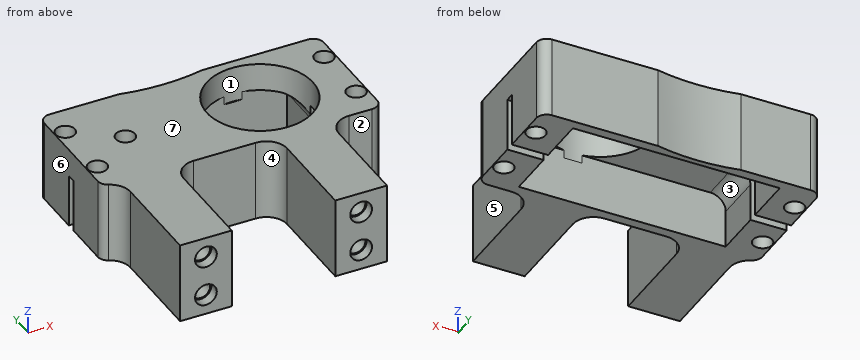
from build123d import *

# Parameters (mm, degrees)
SKETCH035_R                   = 7
SKETCH035_R_2                 = 1.85
PAD021_DEPTH                  = 5.4
PAD021_DEPTH_BACK             = 10.3
POCKET019_DEPTH               = 10.1
SKETCH039_W                   = 1.7
SKETCH039_H                   = 20
POCKET020_DEPTH               = 54.001
SKETCH043_R                   = 10.25
POCKET023_DEPTH               = 7
SKETCH044_W                   = 10
SKETCH044_H                   = 7.85
PAD025_DEPTH                  = 22
SKETCH045_R                   = 1.85
POCKET024_DEPTH               = 12
SKETCH046_R                   = 2.1
POCKET025_DEPTH               = 2
SKETCH044_MIRRORED002_2_W     = 10
SKETCH044_MIRRORED002_2_H     = 7.85
PAD025_MIRRORED002_2_DEPTH    = 22
SKETCH045_MIRRORED002_2_R     = 1.85
POCKET024_MIRRORED002_2_DEPTH = 12
SKETCH046_MIRRORED002_2_R     = 2.1
POCKET025_MIRRORED002_2_DEPTH = 2
FILLET009_R                   = 4


with BuildPart() as part:
    # Sketch035 → Pad021 (new body, two sides)
    with BuildSketch(Plane.XY) as pad021_sk:
        with BuildLine():
            Line((-23.5, 10), (-23.5, -10))
            ThreePointArc((-23.5, -10), (-22.914214, -11.414214), (-21.5, -12))
            Line((-21.5, -12), (28.5, -12))
            ThreePointArc((28.5, -12), (29.914214, -11.414214), (30.5, -10))
            Line((30.5, -10), (30.5, 10))
            ThreePointArc((30.5, 10), (29.914214, 11.414214), (28.5, 12))
            Line((8, 12), (28.5, 12))
            ThreePointArc((-8, 12), (0, 11.167024), (8, 12))
            Line((-21.5, 12), (-8, 12))
            ThreePointArc((-21.5, 12), (-22.914214, 11.414214), (-23.5, 10))
        make_face()
        with Locations((13, 0)):
            Circle(SKETCH035_R, mode=Mode.SUBTRACT)
        with Locations((-21.5, 6)):
            Circle(SKETCH035_R_2, mode=Mode.SUBTRACT)
        with Locations((-21.5, -6)):
            Circle(SKETCH035_R_2, mode=Mode.SUBTRACT)
        with Locations((28.5, 6)):
            Circle(SKETCH035_R_2, mode=Mode.SUBTRACT)
        with Locations((28.5, -6)):
            Circle(SKETCH035_R_2, mode=Mode.SUBTRACT)
        with Locations((-13, 0)):
            Circle(SKETCH035_R_2, mode=Mode.SUBTRACT)
    extrude(amount=PAD021_DEPTH)
    extrude(pad021_sk.sketch, amount=-PAD021_DEPTH_BACK)

    # Sketch038 → Pocket019 (cut, symmetric)
    with BuildSketch(Plane.XZ):
        with BuildLine():
            Line((-16.5, -3), (-16.5, -20))
            Line((-16.5, -20), (23.5, -20))
            Line((23.5, -20), (23.5, -3))
            ThreePointArc((23.5, -3), (22.62132, -0.87868), (20.5, 0))
            Line((20.5, 0), (-13.5, 0))
            ThreePointArc((-13.5, 0), (-15.62132, -0.87868), (-16.5, -3))
        make_face()
    extrude(amount=POCKET019_DEPTH, both=True, mode=Mode.SUBTRACT)

    # Sketch039 (on Face3 of Pocket019) → Pocket020 (cut, through all)
    with BuildSketch(Plane(origin=(-23.5, 0, 0), x_dir=(0, -1, 0), z_dir=(-1, 0, 0))):
        with Locations((0, -10)):
            Rectangle(SKETCH039_W, SKETCH039_H)
    extrude(amount=-POCKET020_DEPTH, mode=Mode.SUBTRACT)

    # Sketch043 (on Face5 of Pocket020) → Pocket023 (cut)
    with BuildSketch(Plane.XY.offset(5.4)):
        with Locations((13, 0)):
            Circle(SKETCH043_R)
    extrude(amount=-POCKET023_DEPTH, mode=Mode.SUBTRACT)

    # Sketch044 → Pad025 (join)
    with BuildSketch(Plane(origin=(0, -12, -2.45), x_dir=(1, 0, 0), z_dir=(0, -1, 0))):
        with Locations((-15, 3.925)):
            Rectangle(SKETCH044_W, SKETCH044_H)
    pad025 = extrude(amount=PAD025_DEPTH)

    # Sketch045 (on Face43 of Pad025) → Pocket024 (cut)
    with BuildSketch(Plane.XZ.offset(34)):
        with Locations((-15, 1.475)):
            Circle(SKETCH045_R)
    pocket024 = extrude(amount=-POCKET024_DEPTH, mode=Mode.SUBTRACT)

    # Sketch046 (on Face43 of Pocket024) → Pocket025 (cut)
    with BuildSketch(Plane.XZ.offset(34)):
        with Locations((-15, 1.475)):
            Circle(SKETCH046_R)
    pocket025 = extrude(amount=-POCKET025_DEPTH, mode=Mode.SUBTRACT)

    # Sketch044 Mirrored002 2 → Pad025 Mirrored002 2 (add)
    with BuildSketch(Plane(origin=(0, -12, -2.45), x_dir=(-1, 0, 0), z_dir=(0, 1, 0))):
        with Locations((-15, 3.925)):
            Rectangle(SKETCH044_MIRRORED002_2_W, SKETCH044_MIRRORED002_2_H)
    pad025_mirrored002_2 = extrude(amount=-PAD025_MIRRORED002_2_DEPTH)

    # Sketch045 Mirrored002 2 → Pocket024 Mirrored002 2 (cut)
    with BuildSketch(Plane(origin=(0, -34, 0), x_dir=(-1, 0, 0), z_dir=(0, 1, 0))):
        with Locations((-15, 1.475)):
            Circle(SKETCH045_MIRRORED002_2_R)
    pocket024_mirrored002_2 = extrude(amount=POCKET024_MIRRORED002_2_DEPTH, mode=Mode.SUBTRACT)

    # Sketch046 Mirrored002 2 → Pocket025 Mirrored002 2 (cut)
    with BuildSketch(Plane(origin=(0, -34, 0), x_dir=(-1, 0, 0), z_dir=(0, 1, 0))):
        with Locations((-15, 1.475)):
            Circle(SKETCH046_MIRRORED002_2_R)
    pocket025_mirrored002_2 = extrude(amount=POCKET025_MIRRORED002_2_DEPTH, mode=Mode.SUBTRACT)

    # Mirrored003: Pad025, Pocket024, Pocket025, Pad025 Mirrored002 2, Pocket024 Mirrored002 2, Pocket025 Mirrored002 2 across Sketch044 H_Axis
    add(pad025.mirror(Plane(origin=(0, -12, -2.45), x_dir=(0, -1, 0), z_dir=(0, 0, 1))))
    add(pocket024.mirror(Plane(origin=(0, -12, -2.45), x_dir=(0, -1, 0), z_dir=(0, 0, 1))), mode=Mode.SUBTRACT)
    add(pocket025.mirror(Plane(origin=(0, -12, -2.45), x_dir=(0, -1, 0), z_dir=(0, 0, 1))), mode=Mode.SUBTRACT)
    add(pad025_mirrored002_2.mirror(Plane(origin=(0, -12, -2.45), x_dir=(0, -1, 0), z_dir=(0, 0, 1))))
    add(pocket024_mirrored002_2.mirror(Plane(origin=(0, -12, -2.45), x_dir=(0, -1, 0), z_dir=(0, 0, 1))), mode=Mode.SUBTRACT)
    add(pocket025_mirrored002_2.mirror(Plane(origin=(0, -12, -2.45), x_dir=(0, -1, 0), z_dir=(0, 0, 1))), mode=Mode.SUBTRACT)

    # Fillet009
    fillet009_edges = [part.edges().sort_by_distance(p)[0] for p in [
        (-20, -12, -2.45),
        (-10, -12, -2.45),
        (10, -12, -2.45),
        (20, -12, -2.45),
    ]]
    fillet(fillet009_edges, radius=FILLET009_R)


with BuildPart() as part_1:
    # Body009 placement: moved
    add(part.part.moved(Location((0, -50, 0))))


solid = part_1.part
Read the model definition and answer for the solid it produces. Units are mm, in the model's axes. Face numbers are marked on the shaded views. A direction names the side the tool comes from. Round coordinates to 2 decimals unless told otherwise and drop trailing zeros. Write each loop counter-clockwise with the first axis right and the second up, starting at its lowest first coordinate (ties: lowest second). Pieces come first, ordered by that corner, then holes.
Q1. Find section C-C on x = -9. Determine the outline of the cut face in (y, z).
Values:
outline: (-63.35, -10.3) - (-60.1, -10.3) - (-60.1, 0) - (-39.9, 0) - (-39.9, -10.3) - (-38, -10.3) - (-38, 5.4) - (-63.35, 5.4) - close
Q2. Find section A-A on y = -69. Determine the outline of the cut face in (x, z), and give its area (3 significant figures).
Values:
outline: (-20, -10.3) - (-10, -10.3) - (-10, 5.4) - (-20, 5.4) - close; (10, -10.3) - (20, -10.3) - (20, 5.4) - (10, 5.4) - close
area: 314 mm2
Q3. A tool of negligible diameter and unlimited length cuts with its end or side. For the marked faces 1, 2 and 3, from which of +Z, -Z, +X, -X, +Y, -Y can it reach the whole face along a straight path? Write none if from no direction.
Values:
face 1: +Z
face 2: +Z, -Z, +X, -Y
face 3: -Z
Q4. Straight lines are drawn through the part: line 1 (X direction, y = -50, z = 4); line 2 (Z direction, x = 15, y = -77) (3 decimals); line 3 (Y direction, x = -13, z = 3.5). For each, find the intervals that lie inside material, in ascending order.
Values:
line 1: x = -23.5 to -14.85, -11.15 to 2.75, 23.25 to 30.5
line 2: z = -10.3 to -8.225, -4.525 to -0.375, 3.325 to 5.4
line 3: y = -84 to -51.85, -48.15 to -38
Q5. Find section B-B on y = -50. Determine the outline of the cut face in (x, z).
Values:
outline: (-23.5, 0) - (-14.85, 0) - (-14.85, 5.4) - (-23.5, 5.4) - close; (-11.15, 0) - (2.75, 0) - (2.75, 5.4) - (-11.15, 5.4) - close; (23.25, 0) - (30.5, 0) - (30.5, 5.4) - (23.25, 5.4) - close
Q6. Flat-ended cylindrical pins translate along their axes: P1, Ø0.9, axis at x = 18, y = -41, coming from the -Z side; P2, Ø1, axis at y = -78.5, z = 3, coming from the +X side; P3, Ø1.1, axis at x = -15.5, z = -6, coming from the -Y side. Find the tip coordinate at first contact, or state that the pin passes through.
Values:
P1: stops at z = 0
P2: stops at x = 20
P3: stops at y = -72
Q7. The mould has two halves that part along X. Classify the marked faces 4, 5, 6 and 7: released by +X, released by -X, zero draft, split by the parting line, or undercut.
Values:
face 4: undercut
face 5: released by +X
face 6: released by -X
face 7: zero draft
